Study the drawing (mm; zero at the part's minimum x, y, z) and answer. A direction names the side the tool comes from. Round coordinates to 2 decimals unless told otherwise and drop trailing zeros. Write each loop counter-clockwise with the first axis right and the second up, starting at its lowest first coordinate (ties: lowest second). Pieces come first, ordered by that corner, then holes. Notation, with made-up numbers: (-6.75, 89.5) -> (13.25, 89.5) arc R25 ccw to (13.25, 111.5) -> close; hole circle Ø11 at (-6, 12.5). An arc over 180 degrees is marked (long way). Return JSON: item names as keys, results as strings.
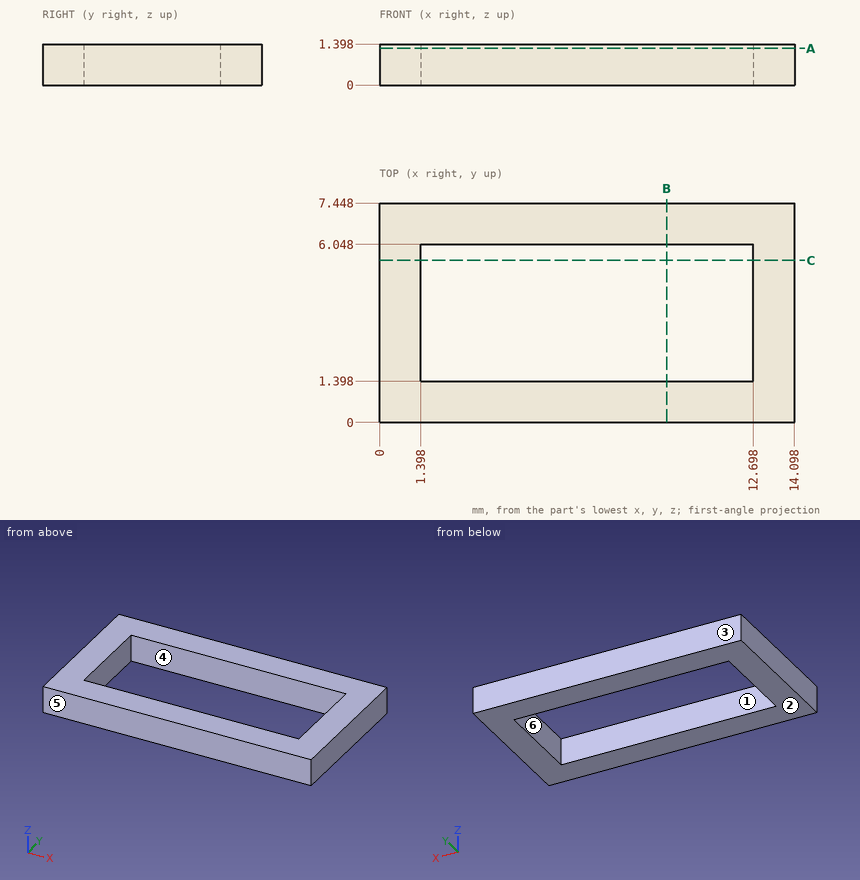
Item 1: Straight lines are drawn through the part: L1, parallel to X at y = 5.25, z = 1.1; L2, parallel to Y at x = 10.75, z = 1.1. For each, find the intervals that lie inside material, in ascending order. Write a range as [from, to].
Worked answers:
{"L1": "x = [0, 1.4], [12.7, 14.1]", "L2": "y = [0, 1.4], [6.05, 7.45]"}
Item 2: Section A-A (z = 1.25) is taken. Give the vertices of the cut face in (x, y), then the cut area to 3 significant figures.
Worked answers:
{"outline": "(0, 0) -> (14.1, 0) -> (14.1, 7.45) -> (0, 7.45) -> close; hole (1.4, 1.4) -> (12.7, 1.4) -> (12.7, 6.05) -> (1.4, 6.05) -> close", "area": "52.5 mm2"}
Item 3: Section C-C (y = 5.5) is taken. Give the vertices of the cut face in (x, z), then the cut area to 3 significant figures.
Worked answers:
{"outline": "(0, 0) -> (1.4, 0) -> (1.4, 1.4) -> (0, 1.4) -> close; (12.7, 0) -> (14.1, 0) -> (14.1, 1.4) -> (12.7, 1.4) -> close", "area": "3.91 mm2"}
Item 4: A tool of negligible diameter and unlimited length cuts with its end or side. For the marked faces 5 and 6, from which of +Z, -Z, +X, -X, +Y, -Y can it reach the whole face along a straight path? Write none if from no direction.
Worked answers:
{"face 5": "+Z, -Z, +X, -X, -Y", "face 6": "+Z, -Z"}
Item 5: Section B-B (x = 9.75) is taken. Give the vertices of the cut face in (y, z).
Worked answers:
{"outline": "(0, 0) -> (1.4, 0) -> (1.4, 1.4) -> (0, 1.4) -> close; (6.05, 0) -> (7.45, 0) -> (7.45, 1.4) -> (6.05, 1.4) -> close"}
Item 6: For a pull along Y with two mould halves and no side action, classify the marked faces 1, 2, 3 and 4 as released by +Y, released by -Y, zero draft, split by the parting line, or undercut.
Worked answers:
{"face 1": "undercut", "face 2": "zero draft", "face 3": "released by +Y", "face 4": "undercut"}
